Could you check a few things on this model? Use its own coordinates, in mm. Face numbers are marked on the shaded views. A direction names the side the tool comes from. Give positions to 0.01 mm unless a question says otherwise; leave off trailing zeros. Loops run counter-clockwise (first coordinate to the right, second up) from the corner with the lowest first, then second, coordinate; pieces in that order, holes last. Notation, with made-up numbers: M 24.25,32.25 L 67.25,32.25 A18 cw 67.25,55.25 Z; hole C 82.5,16.5 d2. An arc over 180 degrees is marked long. Answer in a Markdown table with one row per item. Add a question column.
```python
from build123d import *

# Parameters (mm, degrees)
SKETCH1_W           = 8.4
SKETCH1_H           = 12.6
BOSS_EXTRUDE1_DEPTH = 10.8
CHAMFER1_SIZE       = 1
BOSS_EXTRUDE2_DEPTH = 1.8
SKETCH3_W           = 8.4
SKETCH3_H           = 1.7
CUT_EXTRUDE1_DEPTH  = 8.1
SKETCH4_R           = 1
BOSS_EXTRUDE3_DEPTH = 0.8
SKETCH5_W           = 9
SKETCH5_H           = 3.5
CUT_EXTRUDE2_DEPTH  = 1
SKETCH6_W           = 0.5
SKETCH6_H           = 6.5
BOSS_EXTRUDE4_DEPTH = 0.125


with BuildPart() as part:
    # Sketch1 → Boss-Extrude1 (new body)
    with BuildSketch(Plane.XY):
        with Locations((0, -2.4)):
            Rectangle(SKETCH1_W, SKETCH1_H)
    extrude(amount=BOSS_EXTRUDE1_DEPTH)

    # Chamfer1
    chamfer1_edges = [part.edges().sort_by_distance(p)[0] for p in [
        (-4.2, 3.9, 5.4),
        (4.2, 3.9, 5.4),
    ]]
    chamfer(chamfer1_edges, length=CHAMFER1_SIZE)

    # Sketch2 → Boss-Extrude2 (add)
    with BuildSketch(Plane(origin=(0, 0, 0), x_dir=(-1, 0, 0), z_dir=(0, 0, -1))):
        with BuildLine():
            Line((-7.84, -8.7), (7.84, -8.7))
            ThreePointArc((7.84, -8.7), (9.438061325, -8.038061325), (10.1, -6.44))
            Line((10.1, -6.44), (10.1, -3.96))
            ThreePointArc((10.1, -3.96), (9.438061325, -2.361938675), (7.84, -1.7))
            Line((7.84, -1.7), (-7.84, -1.7))
            ThreePointArc((-7.84, -1.7), (-9.438061325, -2.361938675), (-10.1, -3.96))
            Line((-10.1, -3.96), (-10.1, -6.44))
            ThreePointArc((-10.1, -6.44), (-9.438061325, -8.038061325), (-7.84, -8.7))
        make_face()
        with BuildLine():
            Line((-6.1, -5), (-6.1, -6.4))
            ThreePointArc((-6.1, -6.4), (-7.5, -7.8), (-8.9, -6.4))
            Line((-8.9, -6.4), (-8.9, -5))
            ThreePointArc((-8.9, -5), (-7.5, -3.6), (-6.1, -5))
        make_face(mode=Mode.SUBTRACT)
        with BuildLine():
            Line((8.9, -5), (8.9, -6.4))
            ThreePointArc((8.9, -6.4), (7.5, -7.8), (6.1, -6.4))
            Line((6.1, -6.4), (6.1, -5))
            ThreePointArc((6.1, -5), (7.5, -3.6), (8.9, -5))
        make_face(mode=Mode.SUBTRACT)
    extrude(amount=-BOSS_EXTRUDE2_DEPTH)

    # Sketch3 → Cut-Extrude1 (cut)
    with BuildSketch(Plane(origin=(0, 3.9, 0), x_dir=(1, 0, 0), z_dir=(0, 1, 0))):
        with Locations((0, -4.75)):
            Rectangle(SKETCH3_W, SKETCH3_H)
    extrude(amount=-CUT_EXTRUDE1_DEPTH, mode=Mode.SUBTRACT)

    # Sketch4 → Boss-Extrude3 (add)
    with BuildSketch(Plane(origin=(0, 0, 0), x_dir=(-1, 0, 0), z_dir=(0, 0, -1))):
        Circle(SKETCH4_R)
        with Locations((0, -6.4)):
            Circle(SKETCH4_R)
    extrude(amount=BOSS_EXTRUDE3_DEPTH)

    # Sketch5 → Cut-Extrude2 (cut)
    with BuildSketch(Plane.XZ.offset(8.7)):
        with Locations((0, 1.75)):
            Rectangle(SKETCH5_W, SKETCH5_H)
    extrude(amount=-CUT_EXTRUDE2_DEPTH, mode=Mode.SUBTRACT)

    # Sketch6 → Boss-Extrude4 (add, symmetric)
    with BuildSketch(Plane(origin=(0, 0, 3), x_dir=(-1, 0, 0), z_dir=(0, 0, -1))):
        with Locations((-3.81, -10.95)):
            Rectangle(SKETCH6_W, SKETCH6_H)
        with Locations((-1.27, -10.95)):
            Rectangle(SKETCH6_W, SKETCH6_H)
        with Locations((1.27, -10.95)):
            Rectangle(SKETCH6_W, SKETCH6_H)
        with Locations((3.81, -10.95)):
            Rectangle(SKETCH6_W, SKETCH6_H)
    extrude(amount=BOSS_EXTRUDE4_DEPTH, both=True)


solid = part.part
```
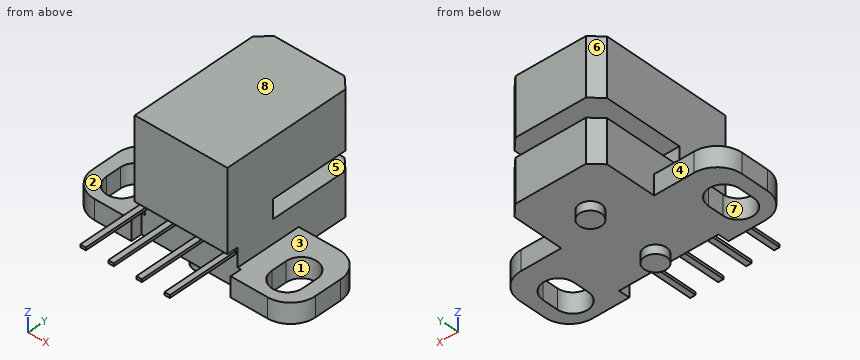
Item 1: For the marked faces 1, 2, 3, 4 and 5, which set-ups out of +Z, -Z, +X, -X, +Y, -Y let a thin tool reach every point of the face, with its end or its side?
Item 2: Suppose I cut it at D-D (x = 0). List the corners of the cut face in (y, z) for me, then the cut area to 3 significant figures.
Item 3: I need wall thicknesses on L1, parallel to Z at x = 1.5, y = 1.25; L2, parallel to X at y = -2.25, z = 6.75; L3, parallel to Y at x = 0.75, z = 2.25. Which ranges of each line are inside material? Lowest first, please.
Item 4: For P1, Ø6, axis at x = 3, y = -5.5, coming from the -Z side; P2, Ø0.6, axis at x = -1, y = -11, coming from the +Z side (3 decimals); P3, Ø1.1, axis at x = 1.5, y = -8.5, coming from the -Z side (3 decimals); P4, Ø6, axis at y = -1.5, z = 8, coming from the -X side, each with a flat end and sliding along its axis, tell me the tip position at first contact or that it passes through.
Item 5: Suppose I cut it at B-B (y = -12). List the corners of the cut face in (x, z) for me (3 decimals).
Item 6: Suppose I cut it at A-A (x = 7.5). List the corners of the cut face in (y, z) for me.
Item 7: If we mould it in two halves opening along X, with no side actions, what happens to the marked faces 6, 7 and 8? For each: +X half, -X half, draft (parallel to the pull), parting line (faces both ways), or undercut.
Item 8: Suppose I cut it at C-C (y = 1.25). List the corners of the cut face in (x, z) for me.
Values found:
| question | item | result |
|---|---|---|
| 1 | face 1 | +Z, -Z |
| 1 | face 2 | +Z, -X, +Y, -Y |
| 1 | face 3 | +Z, +X, +Y, -Y |
| 1 | face 4 | +Z, -Z, -X, +Y |
| 1 | face 5 | +X, -X, +Y |
| 2 | outline | M -8.7,3.5 L -7.7,3.5 L -7.7,0 L -7.4,0 L -7.4,-0.8 L -5.4,-0.8 L -5.4,0 L -1,0 L -1,-0.8 L 1,-0.8 L 1,0 L 3.9,0 L 3.9,3.9 L -4.2,3.9 L -4.2,5.6 L 3.9,5.6 L 3.9,10.8 L -8.7,10.8 Z |
| 2 | area | 122 mm² |
| 3 | L1 | 0 to 3.9, 5.6 to 10.8 |
| 3 | L2 | -4.2 to 4.2 |
| 3 | L3 | -7.7 to 3.9 |
| 4 | P1 | z = -0.8 |
| 4 | P2 | z = 3.125 |
| 4 | P3 | z = 2.875 |
| 4 | P4 | x = -4.2 |
| 5 | outline | M -4.06,2.875 L -3.56,2.875 L -3.56,3.125 L -4.06,3.125 Z; M -1.52,2.875 L -1.02,2.875 L -1.02,3.125 L -1.52,3.125 Z; M 1.02,2.875 L 1.52,2.875 L 1.52,3.125 L 1.02,3.125 Z; M 3.56,2.875 L 4.06,2.875 L 4.06,3.125 L 3.56,3.125 Z |
| 6 | outline | M -8.7,0 L -7.8,0 L -7.8,1.8 L -8.7,1.8 Z; M -3.6,0 L -1.7,0 L -1.7,1.8 L -3.6,1.8 Z |
| 7 | face 6 | -X half |
| 7 | face 7 | undercut |
| 7 | face 8 | draft |
| 8 | outline | M -4.2,0 L 4.2,0 L 4.2,3.9 L -4.2,3.9 Z; M -4.2,5.6 L 4.2,5.6 L 4.2,10.8 L -4.2,10.8 Z |
